```python
from build123d import *

# Parameters (mm, degrees)
F0_W     = 113
F0_H     = 64
F1_DEPTH = 16
F2_W     = 25
F2_H     = 51
F2_H_2   = 34
F2_W_2   = 35
F2_H_3   = 17
F3_DEPTH = 32.001
F4_R     = 6.5
F5_DEPTH = 88.001
F7_R     = 5.5
F8_DEPTH = 64.001
F9_SIZE  = 10


with BuildPart() as f1:
    # F0 (on Front) → F1 (new body, symmetric)
    with BuildSketch(Plane.XZ):
        with Locations((0, 32)):
            Rectangle(F0_W, F0_H)
    extrude(amount=F1_DEPTH, both=True)

    # F2 (on face) → F3 (cut, through all)
    with BuildSketch(Plane.XZ.offset(16)):
        with Locations((-44, 38.5)):
            Rectangle(F2_W, F2_H)
        with Locations((44, 38.5)):
            Rectangle(F2_W, F2_H)
        with Locations((0, 47)):
            Rectangle(F2_W, F2_H_2)
        with Locations((0, 8.5)):
            Rectangle(F2_W_2, F2_H_3)
    extrude(amount=-F3_DEPTH, mode=Mode.SUBTRACT)

    # F4 (on face) → F5 (cut, through all)
    with BuildSketch(Plane.YZ.offset(31.5)):
        with BuildLine():
            ThreePointArc((-16, 60.1287648325), (-8.2308332161, 63.0184271325), (0, 64))
            Line((0, 64), (-16, 64))
            Line((-16, 64), (-16, 60.1287648325))
        make_face()
        with BuildLine():
            ThreePointArc((0, 64), (8.230833216, 63.0184271325), (16, 60.1287648325))
            Line((16, 60.1287648325), (16, 64))
            Line((16, 64), (0, 64))
        make_face()
        with Locations((0, 46)):
            Circle(F4_R)
    extrude(amount=-F5_DEPTH, mode=Mode.SUBTRACT)

    # F7 (on offset) → F8 (cut, through all)
    with BuildSketch(Plane.XY.offset(64)):
        with Locations((-43.5, 3)):
            Circle(F7_R)
        with Locations((43.5, 3)):
            Circle(F7_R)
    extrude(amount=-F8_DEPTH, mode=Mode.SUBTRACT)

    # F9
    f9_edges = [f1.edges().sort_by_distance(p)[0] for p in [
        (56.5, -16, 6.5),
        (-56.5, -16, 6.5),
    ]]
    chamfer(f9_edges, length=F9_SIZE)


solid = f1.part
```
Here's how the part is built. I have some questions about the finished solid (model axes, mm). A direction names the side the tool comes from. Round coordinates to 2 decimals unless told otherwise and drop trailing zeros. Order: outer loops, then holes, each group sorted by start corner. A loop starts at its lowest first (then second) coordinate and runs counter-clockwise, first axis right, second up. Notation, with made-up numbers: M -9.75,40.25 L 2.25,40.25 A20 cw 2.25,71.25 Z; hole C 17,39 d10. An arc over 180 degrees is marked long. One line per question, with ' | ' between items.
1) I want a section at A-A, the plane z = 15.5. Write out the boundary of the cut face in (x, y).
Working result:
outline: M -31.5,-16 L -17.5,-16 L -17.5,16 L -31.5,16 Z; M 17.5,-16 L 31.5,-16 L 31.5,16 L 17.5,16 Z
2) I want a section at C-C, the plane x = -43.5. Write out the boundary of the cut face in (y, z).
Working result:
outline: M -16,0 L -2.5,0 L -2.5,13 L -16,13 Z; M 8.5,0 L 16,0 L 16,13 L 8.5,13 Z
3) For faces 5 (the face through (44, -4, 13)), 6 (the face through (-31.5, 0, 38)), 7 (the face through (0, 0, 30)), which set-ups out of +Z, -Z, +X, -X, +Y, -Y let a thin tool reach every point of the face, with its end or its side?
Working result:
face 5: +Z, +X, +Y, -Y | face 6: +Z, -X, +Y, -Y | face 7: +Z, +Y, -Y
4) I want a section at B-B, the plane z = 46. Write out the boundary of the cut face in (x, y), then the cut area to 3 significant figures.
Working result:
outline: M -31.5,-16 L -12.5,-16 L -12.5,-6.5 L -31.5,-6.5 Z; M -31.5,6.5 L -12.5,6.5 L -12.5,16 L -31.5,16 Z; M 12.5,-16 L 31.5,-16 L 31.5,-6.5 L 12.5,-6.5 Z; M 12.5,6.5 L 31.5,6.5 L 31.5,16 L 12.5,16 Z | area: 722 mm²
5) If we mould it in two halves opening along X, with no side actions, what happens to faces 1 (the face through (56.5, 5, 6)), 2 (the face through (-51.4, -11.1, 6.4)), 3 (the face through (0, 0, 17)), 4 (the face through (22.133, -1.409, 39.655))? For each: +X half, -X half, draft (parallel to the pull), parting line (faces both ways), or undercut.
Working result:
face 1: +X half | face 2: -X half | face 3: undercut | face 4: draft
6) I need wall thicknesses on line 1 along X through (y, z) = (2, 36.5); line 2 along X through (y, z) = (-5, 14.5); line 3 along X through (y, z) = (6.5, 11). Which ranges of each line are inside material? Lowest first, please.
Working result:
line 1: -31.5 to -12.5, 12.5 to 31.5 | line 2: -31.5 to -17.5, 17.5 to 31.5 | line 3: -56.5 to -47.74, -39.26 to -17.5, 17.5 to 39.26, 47.74 to 56.5
7) I want a section at D-D, the plane y = 3. State how many separate pieces and enclosed holes the cut face has, then the cut area to 3 significant figures.
Working result:
separate pieces: 5 | enclosed holes: 0 | area: 2,510 mm²
8) For pin 1 Ø3 at (y, z) = (-4, 16) entering from -X; pin 2 Ø6 at (y, z) = (8.5, 33) entering from +X; pin 3 Ø10.5 at (y, z) = (0, 46) entering from +X; pin 4 Ø14.5 at (x, y) = (43.5, 3) entering from +Z, each with a flat end and sliding along its axis, tell me the tip position at first contact or that it passes through.
Working result:
pin 1: x = -31.5 | pin 2: x = 31.5 | pin 3: through | pin 4: z = 13
